```python
from build123d import *

# Parameters (mm, degrees)
SKETCH2_R           = 1.5
BOSS_EXTRUDE1_DEPTH = 100
BOSS_EXTRUDE2_DEPTH = 3


with BuildPart() as part:
    # Sketch2 → Boss-Extrude1 (new body)
    with BuildSketch(Plane(origin=(0, 0, 0), x_dir=(1, 0, 0), z_dir=(0, 1, 0))):
        Circle(SKETCH2_R)
    extrude(amount=BOSS_EXTRUDE1_DEPTH)

    # Sketch3 → Boss-Extrude2 (add)
    with BuildSketch(Plane(origin=(0, 100, 0), x_dir=(1, 0, 0), z_dir=(0, 1, 0))):
        Polygon((-2.305280672, -0.137892556), (-1.03322188, -2.065377903), (1.272058792, -1.927485347), (2.305280672, 0.137892556), (1.03322188, 2.065377903), (-1.272058792, 1.927485347), align=None)
    extrude(amount=BOSS_EXTRUDE2_DEPTH)


solid = part.part
```
For this review, take the finished solid that the model builds, in its own axes (mm). A direction names the side the tool comes from. Coordinates: 2 decimals unless noted, no trailing zeros. Loops run counter-clockwise (first coordinate to the right, second up) from the corner with the lowest first, then second, coordinate; pieces in that order, holes last.
1. Add section C-C, the plane x = 0. Give the boundary of the cut face in (y, z), then the cut area to 3 significant figures.
2. For faces 1 (the flat face through (0, 0, 0)), 2 (the flat face through (2, 100, 0)), list the 3-axis set-ups (+Z, -Z, +X, -X, +Y, -Y) from which the entire face can be reached by the end or side of a thin tool; tool diameter is ignored.
3. Insertion check: P1, Ø2, axis at x = -1, y = 81.5, coming from the +Z side; P2, Ø2, axis at x = 0, y = 71.5, coming from the -Z side. Each pin has a flat end and moves straight along its axis. Give the tip position at first contact, or say it passes through.
4. Add section A-A, the plane z = 0.85. Give the boundary of the cut face in (x, y), then the cut area to 3 significant figures.
5. Add section B-B, the plane y = 70. Give the boundary of the cut face in (x, z).
6. For line 1 (X direction, y = 94, z = -0.2); line 2 (Z direction, x = 0, y = 29.5); line 3 (Y direction, x = -2.05, z = -0.05), list the stretches that pass through material, from the lowest coordinate up.
Result:
1. outline: (0, -1.5) - (100, -1.5) - (100, -2) - (103, -2) - (103, 2) - (100, 2) - (100, 1.5) - (0, 1.5) - close
1. area: 312 mm2
2. face 1: +Z, -Z, +X, -X, -Y
2. face 2: -Y
3. P1: stops at z = 1.5
3. P2: stops at z = -1.5
4. outline: (-1.84, 100) - (-1.24, 100) - (-1.24, 0) - (1.24, 0) - (1.24, 100) - (1.81, 100) - (1.81, 103) - (-1.84, 103) - close
4. area: 258 mm2
5. outline: circle Ø3 at (0, 0)
6. line 1: x = -1.49 to 1.49
6. line 2: z = -1.5 to 1.5
6. line 3: y = 100 to 103
